Autodesk Fusion 360 part; units mm, degrees
sketch "Sketch2" plane through (0, 0, 0) normal (0, 1, 0) x (1, 0, 0)
  line L0 (0, 0) -> (150, 0)
  line L1 (150, 0) -> (150, 50)
  line L2 (150, 50) -> (0, 50)
  line L3 (0, 50) -> (0, 0)
  dimension "d11" = 150
  dimension "d12" = 50
extrude "Extrude2" add sketch "Sketch2" along normal blind 50
fillet "Fillet3" radius 25 4 edges at (0, 50, -25) (0, 0, -25) (150, 50, -25) (150, 0, -25)
sketch "Sketch3" plane through (0, 0, 0) normal (0, 0, 1) x (1, 0, 0)
  arc A0 (125, 0) -> (125, 50) centre (125, 25) ccw
  line L0 (125, 50) -> (25, 50)
  arc A1 (25, 50) -> (25, 0) centre (25, 25) ccw
  line L1 (25, 0) -> (125, 0)
  circle A2 centre (20, 25) radius 12
  circle A3 centre (130, 25) radius 12
  dimension "d19" = 24
  dimension "d20" = 24
extrude "Extrude3" cut sketch "Sketch3" against normal blind 105 contours A2 | A3
sketch "Sketch4" plane through (0, 0, 0) normal (0, 0, 1) x (1, 0, 0)
  line L0 (110.0001, 14.8) -> (89.6001, 14.8)
  line L1 (89.6001, 14.8) -> (89.6001, 35.2)
  line L2 (89.6001, 35.2) -> (110.0001, 35.2)
  line L3 (110.0001, 35.2) -> (110.0001, 14.8)
  line L4 (40, 35.2) -> (60.4, 35.2)
  line L5 (60.4, 35.2) -> (60.4, 14.8)
  line L6 (60.4, 14.8) -> (40, 14.8)
  line L7 (40, 14.8) -> (40, 35.2)
extrude "Extrude4" cut sketch "Sketch4" against normal blind 25
sketch "Sketch5" plane through (0, 0, 0) normal (0, 0, 1) x (1, 0, 0)
  line L0 (60.4, 35.2) -> (60.4, 14.8)
  line L1 (60.4, 14.8) -> (40, 14.8)
  line L2 (40, 14.8) -> (40, 35.2)
  line L3 (40, 35.2) -> (60.4, 35.2)
  line L4 (89.6001, 14.8) -> (89.6001, 35.2)
  line L5 (89.6001, 35.2) -> (110.0001, 35.2)
  line L6 (110.0001, 35.2) -> (110.0001, 14.8)
  line L7 (110.0001, 14.8) -> (89.6001, 14.8)
  circle A0 centre (20, 25) radius 12
  circle A1 centre (130, 25) radius 12
  arc A2 (125, 0) -> (125, 50) centre (125, 25) ccw
  line L8 (125, 50) -> (25, 50)
  arc A3 (25, 50) -> (25, 0) centre (25, 25) ccw
  line L9 (25, 0) -> (125, 0)
  circle A4 centre (50.2, 25) radius 2.5
  circle A5 centre (99.8001, 25) radius 2.5
  dimension "d39" = 5
  dimension "d40" = 5
extrude "Extrude5" cut sketch "Sketch5" against normal blind 85 contours A4 | A5
sketch "Sketch6" plane through (0, 0, 0) normal (0, 0, 1) x (1, 0, 0)
  circle A0 centre (50.2, 25) radius 8
  circle A1 centre (99.8, 25) radius 8
  dimension "d43" = 16
  dimension "d44" = 16
extrude "Extrude6" cut sketch "Sketch6" against normal blind 26
sketch "Sketch7" plane through (0, 0, 0) normal (0, 0, 1) x (1, 0, 0)
  line L0 (60.4, 35.2) -> (60.4, 14.8)
  line L1 (60.4, 14.8) -> (40, 14.8)
  line L2 (40, 14.8) -> (40, 35.2)
  line L3 (40, 35.2) -> (60.4, 35.2)
  line L4 (89.6001, 14.8) -> (89.6001, 35.2)
  line L5 (89.6001, 35.2) -> (110.0001, 35.2)
  line L6 (110.0001, 35.2) -> (110.0001, 14.8)
  line L7 (110.0001, 14.8) -> (89.6001, 14.8)
  circle A0 centre (20, 25) radius 12
  circle A1 centre (130, 25) radius 12
  arc A2 (125, 0) -> (125, 50) centre (125, 25) ccw
  line L8 (125, 50) -> (25, 50)
  arc A3 (25, 50) -> (25, 0) centre (25, 25) ccw
  line L9 (25, 0) -> (125, 0)
  circle A4 centre (42.1991, 33.0009) radius 1.1
  circle A5 centre (58.2009, 33.0009) radius 1.1
  circle A6 centre (58.2009, 16.9991) radius 1.1
  circle A7 centre (42.1991, 16.9991) radius 1.1
  circle A8 centre (91.7992, 33.001) radius 1.1
  circle A9 centre (91.7992, 16.999) radius 1.1
  circle A10 centre (107.801, 16.9992) radius 1.1
  circle A11 centre (107.801, 33.0008) radius 1.1
  dimension "d48" = 2.2
  dimension "d49" = 2.2
  dimension "d50" = 2.2
  dimension "d51" = 2.2
  dimension "d53" = 2.2
  dimension "d54" = 2.2
  dimension "d55" = 2.2
  dimension "d56" = 2.2
sketch "Sketch8" plane through (0, 0, -50) normal (0, 0, -1) x (-1, 0, 0)
  circle A0 centre (-50.2, 25) radius 2.5
  circle A1 centre (-99.8001, 25) radius 2.5
  circle A2 centre (-20, 25) radius 12
  circle A3 centre (-130, 25) radius 12
  arc A4 (-125, 50) -> (-125, 0) centre (-125, 25) ccw
  line L0 (-125, 0) -> (-25, 0)
  arc A5 (-25, 0) -> (-25, 50) centre (-25, 25) ccw
  line L1 (-25, 50) -> (-125, 50)
  line L2 (-107.801, 16.9992) -> (-105.9894, 15.4871)
  curve L3
  curve L4
  curve L5
  curve L6
  line L7 (-91.7992, 16.999) -> (-88.5659, 15.2744)
  line L8 (-58.2009, 33.0009) -> (-55, 31)
  line L9 (-42.1991, 33.0009) -> (-38, 28)
  line L10 (-58.2009, 16.9991) -> (-57, 14)
  line L11 (-42.1991, 16.9991) -> (-41, 14)
  dimension "d60" = 6.53
hole "Hole1" at (107.801, 33.0008, -50) at (91.7992, 33.001, -50) at (91.7992, 16.999, -50) at (107.801, 16.9992, -50) at (58.2009, 16.9991, -50) at (58.2009, 33.0009, -50) at (42.1991, 33.0009, -50) at (42.1991, 16.9991, -50) direction (0, 0, 1) diameter 1.775 depth 35 tip angle 118 counterbore diameter 4 counterbore depth 2
Model file for the job. Use its own axes, mm. A direction names the side the tool comes from. Round coordinates to 2 decimals unless told otherwise and drop trailing zeros. Order: outer loops, then holes, each group sorted by start corner. A loop starts at its lowest first (then second) coordinate and runs counter-clockwise, first axis right, second up. Notation, with made-up numbers: M 82.5,-22.75 L 119.5,-22.75 A21 cw 119.5,-7.75 Z; hole C -26.5,66.25 d6. An arc over 180 degrees is marked long. Write each question's results on one line, items separated by ' | '. Start each with the question number.
(1) Saw through at D-D, the plane x = 20. Give the cut face in (y, z), then the cut area to 3 significant figures.
(2) Drop flat-ended pins along their axis: pin 1 (6 mm diameter, centred on x = 98, z = -12, fed in from -Y); pin 2 (1.5 mm diameter, centred on y = 14.5, z = -14, fed in from -X); pin 3 (3 mm diameter, centred on x = 107.8, y = 17, fed in from +Z); pin 4 (1.5 mm diameter, centred on y = 29.5, z = -11.5, fed in from -X). Give the stop position or say it passes through.
(3) Probe probe 1 along X at (y, z) = (33, -20.5); probe 2 along X at (y, z) = (35, -7); probe 3 along X at (y, z) = (20.5, -44.5). List the from-to ranges inside material, lowest first. Write a range as from..to.
(4) Saw through at B-B, the plane y = 29. Give the cut face in (x, z).
(5) Which spindle directions (+Z, -Z, +X, -X, +Y, -Y) get a long thin tool onto all of the face, cutting with end or side? Do faces 1 (the face through (56.22, 32.74, -48.99)), 2 (the face through (7.128, 7.516, -24.65)), 3 (the face through (93, 30, -25)). Say none if no direction does.
(6) Saw through at A-A, the plane x = 50.2. Give the cut face in (y, z).
(7) Two-plate mould, pull along X, no slides. Class faces 4 (the face through (74, 0, -25)), 5 (the face through (50, 14.8, -12)), 6 (the face through (142.872, 7.516, -25.35)): pulls with the +X half, pulls with the -X half, needs draft (parallel to the pull), parting line crosses it, or undercut.
(8) Saw through at C-C, the plane z = -35. State how many separate pieces and enclosed holes the cut face has, then the cut area to 3 significant figures.
Established:
1) outline: M 0.5,-50 L 13,-50 L 13,0 L 0.5,0 Z; M 37,-50 L 49.5,-50 L 49.5,0 L 37,0 Z | area: 1,250 mm^2
2) pin 1: stops at y = 0 | pin 2: stops at x = 1.98 | pin 3: stops at z = -25 | pin 4: stops at x = 0.28
3) probe 1: x = 1.31..11.06, 28.94..40, 60.4..89.6, 110..121.06, 138.94..148.69 | probe 2: x = 2.09..13.37, 26.63..40, 60.4..89.6, 110..123.37, 136.63..147.91 | probe 3: x = 0.41..8.88, 31.12..118.88, 141.12..149.59
4) outline: M 0.32,-50 L 8.69,-50 L 8.69,0 L 0.32,0 Z; M 31.31,-50 L 118.69,-50 L 118.69,0 L 110,0 L 110,-25 L 106.73,-25 L 106.73,-26 L 92.87,-26 L 92.87,-25 L 89.6,-25 L 89.6,0 L 60.4,0 L 60.4,-25 L 57.13,-25 L 57.13,-26 L 43.27,-26 L 43.27,-25 L 40,-25 L 40,0 L 31.31,0 Z; M 141.31,-50 L 149.68,-50 L 149.68,0 L 141.31,0 Z
5) face 1: -Z | face 2: +Z, -Z, -X, -Y | face 3: +Z
6) outline: M 0,-50 L 22.5,-50 L 22.5,-26 L 17,-26 L 17,-25 L 14.8,-25 L 14.8,0 L 0,0 Z; M 27.5,-50 L 50,-50 L 50,0 L 35.2,0 L 35.2,-25 L 33,-25 L 33,-26 L 27.5,-26 Z
7) face 4: needs draft | face 5: undercut | face 6: pulls with the +X half
8) separate pieces: 1 | enclosed holes: 12 | area: 6,000 mm^2
